from build123d import *

# Parameters (mm, degrees)
BASE_FLANGE1_DEPTH     = 1.524
SKETCHED_START         = -12.348324115
SKETCHED_BEND6_DEPTH   = 24.69664823
SKETCHED_BEND6_2_DEPTH = 24.69664823


# Read off the part's stored shape, not the designer's step: Sketched Bend6
# Sheet-metal steps are written as plain solids
with BuildPart() as part:
    # Sketch2 → Base-Flange1 (new body)
    with BuildSketch(Plane(origin=(0, 0, 0), x_dir=(1, 0, 0), z_dir=(0, 1, 0))):
        Polygon((12.348324115, -35), (12.348324115, 35), (12.348324115, 45), (-12.348324115, 45), (-12.348324115, 35), (-12.348324115, -35), align=None)
    extrude(amount=-BASE_FLANGE1_DEPTH)

    # Sketched Bend6 outline → Sketched Bend6 (cut)
    with BuildSketch(Plane.YZ.offset(SKETCHED_START)):
        with BuildLine():
            Line((0, -45), (0, -34.876625492))
            ThreePointArc((0, -34.876625492), (-1.103980115, -34.051869886), (-1.524, -32.7394))
            Line((-1.524, -32.7394), (-1.524, -45))
            Line((-1.524, -45), (0, -45))
        make_face()
    extrude(amount=SKETCHED_BEND6_DEPTH, mode=Mode.SUBTRACT)

    # Sketched Bend6 2 outline → Sketched Bend6 2 (add)
    with BuildSketch(Plane.YZ.offset(SKETCHED_START)):
        with BuildLine():
            Line((10.643204625, -33.476), (0.7366, -33.476))
            ThreePointArc((0.7366, -33.476), (0.215745145, -33.260254855), (0, -32.7394))
            Line((0, -32.7394), (0, -34.876625492))
            ThreePointArc((0, -34.876625492), (0.363169675, -34.968943037), (0.7366, -35))
            Line((0.7366, -35), (10.643204625, -35))
            Line((10.643204625, -35), (10.643204625, -33.476))
        make_face()
    extrude(amount=SKETCHED_BEND6_2_DEPTH)


solid = part.part
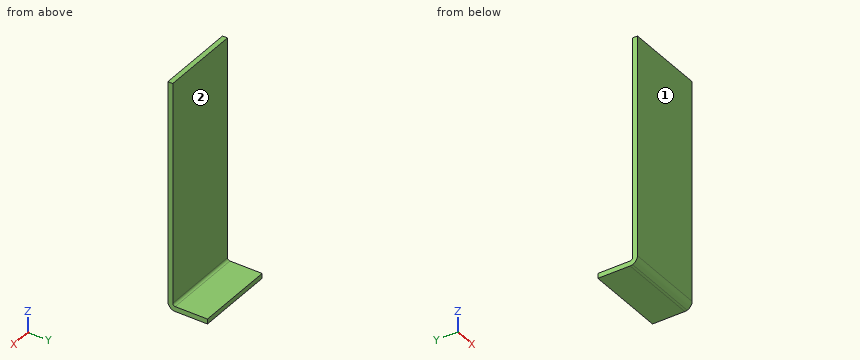
Geometry: final body of the model. Coordinates: model frame, mm. Face numbers are marked on the shaded views. A direction names the side the tool comes from. Round coordinates to 2 decimals unless told otherwise and drop trailing zeros. Loops run counter-clockwise (first coordinate to the right, second up) from the corner with the lowest first, then second, coordinate; pieces in that order, holes last. Notation, with made-up numbers: M 53,1 L 108,1 A28 cw 108,28 Z; hole C -22,83.5 d3. An arc over 180 degrees is marked long. One line per question, with ' | ' between items.
(1) Material intervals for line 1 along Y through (x, z) = (-5.5, -7.5); line 2 along Z through (x, y) = (1.5, 1), sorted ascending. Write a range as from..to.
Check result:
line 1: y = -1.52..0 | line 2: z = -35..-33.48
(2) Cut plane C-C on y = 2.25. Return the cut outline in (x, z), plus the area to 3 significant figures.
Check result:
outline: M -12.35,-35 L 12.35,-35 L 12.35,-33.48 L -12.35,-33.48 Z | area: 37.6 mm2
(3) Contact query for flat-ended pins moving along their axis: P1, Ø12.5, axis at x = -1, z = 11, coming from the +Y side; P2, Ø6, axis at x = 1.5, y = 7.5, coming from the +Z side; P3, Ø6, axis at y = 4, z = -20.5, coming from the -X side. Output: stop coordinate, or through.
Check result:
P1: stops at y = 0 | P2: stops at z = -33.48 | P3: passes through
(4) Cut plane B-B on z = 24. Return the cut outline in (x, y).
Check result:
outline: M -12.35,-1.52 L 12.35,-1.52 L 12.35,0 L -12.35,0 Z
(5) Access query for the marked faces 1 and 2. Directions: +Z, -Z, +X, -X, +Y, -Y. A direction counts if a zero-diameter tool reaches every point of the face in a straight line with its end or side. Return the directions, or none.
Check result:
face 1: +Z, -Z, +X, -X, -Y | face 2: +Z, +X, -X, +Y
(6) Cut plane A-A on x = 1.25. Return the cut outline in (y, z).
Check result:
outline: M -1.52,-32.74 A2.26 ccw 0.74,-35 L 10.64,-35 L 10.64,-33.48 L 0.74,-33.48 A0.74 cw 0,-32.74 L 0,35 L -1.52,35 Z
